Source: CAD feature listing. Evaluate the final solid. Frame: model axes, mm. Face numbers are marked on the shaded views. Round coordinates to 2 decimals unless told otherwise and drop trailing zeros. Write each loop counter-clockwise with the first axis right and the second up, starting at its lowest first coordinate (ties: lowest second). Pieces come first, ordered by that corner, then holes. Notation, with made-up numbers: M -37,71 L 1,71 A17 cw 1,84 Z; hole C -38,83.25 d7. An arc over 180 degrees is marked long. Answer in a Markdown table with one row per item. Add a question column.
Item 1: Cut plane D-D on x = -15. Return loops of the section in (y, z), and give its area (3 significant figures).
Item 2: Cut plane C-C on x = -21.75. Return loops of the section in (y, z).
Item 3: Material intervals for probe 1 along Z at (x, y) = (-17, 3.3); probe 2 along X at (y, z) = (4.3, -16); probe 3 along Z at (x, y) = (-12.75, 1.55), sorted ascending.
Item 4: Cut plane B-B on z = -15. Return loops of the section in (x, y).
Item 5: Mould query, pull axis Z, two halves, no side actions, for the marked faces 1, 2 and 3. Classes: released by +Z, released by -Z, zero draft, split by the parting line, or undercut.
Item 6: Contact query for flat-ended pins moving along their axis: pin 1 (5 mm diameter, centred on x = -22.39, z = 15.97, fed in from +Y); pin 2 (3 mm diameter, centred on y = 2.5, z = -20.5, fed in from -X). Output: stop coordinate, or through.
Item 7: Cut plane A-A on y = 4.4. Return loops of the section in (x, z), and give its area (3 significant figures).
from build123d import *

# Parameters (mm, degrees)
SKETCH_1_R          = 15.5
SKETCH_1_R_2        = 1.55
EXTRUDE_1_DEPTH     = 5
SKETCH_3_W          = 44.726871009
SKETCH_3_H          = 71.780776613
CUT_EXTRUDE_2_DEPTH = 10
FILLET_1_R          = 2
FILLET_2_R          = 5


with BuildPart() as part:
    # 草图1 → 凸台-拉伸1 (new body)
    with BuildSketch(Plane(origin=(0, 0, 0), x_dir=(1, 0, 0), z_dir=(0, 1, 0))):
        with BuildLine():
            Line((-17.783419244, 26), (17.783419244, 26))
            ThreePointArc((17.783419244, 26), (22.273863607, 22.273863607), (26, 17.783419244))
            Line((26, 17.783419244), (26, -17.783419244))
            ThreePointArc((26, -17.783419244), (22.273863607, -22.273863607), (17.783419244, -26))
            Line((17.783419244, -26), (-17.783419244, -26))
            ThreePointArc((-17.783419244, -26), (-22.273863607, -22.273863607), (-26, -17.783419244))
            Line((-26, -17.783419244), (-26, 17.783419244))
            ThreePointArc((-26, 17.783419244), (-22.273863607, 22.273863607), (-17.783419244, 26))
        make_face()
        with Locations(Location((0, 0, 0), (0, 0, 270))):
            Circle(SKETCH_1_R, mode=Mode.SUBTRACT)
        with Locations(Location((-22.388176755, 15.969331282, 0), (0, 0, 270))):
            Circle(SKETCH_1_R_2, mode=Mode.SUBTRACT)
        with Locations(Location((-15.969331282, 22.388176755, 0), (0, 0, 90))):
            Circle(SKETCH_1_R_2, mode=Mode.SUBTRACT)
        with Locations(Location((22.388176755, 15.969331282, 0), (0, 0, 90))):
            Circle(SKETCH_1_R_2, mode=Mode.SUBTRACT)
        with Locations(Location((15.969331282, 22.388176755, 0), (0, 0, 270))):
            Circle(SKETCH_1_R_2, mode=Mode.SUBTRACT)
        with Locations(Location((22.388176755, -15.969331282, 0), (0, 0, 270))):
            Circle(SKETCH_1_R_2, mode=Mode.SUBTRACT)
        with Locations(Location((15.969331282, -22.388176755, 0), (0, 0, 90))):
            Circle(SKETCH_1_R_2, mode=Mode.SUBTRACT)
        with Locations(Location((-22.388176755, -15.969331282, 0), (0, 0, 90))):
            Circle(SKETCH_1_R_2, mode=Mode.SUBTRACT)
        with Locations(Location((-15.969331282, -22.388176755, 0), (0, 0, 270))):
            Circle(SKETCH_1_R_2, mode=Mode.SUBTRACT)
    extrude(amount=EXTRUDE_1_DEPTH)

    # 草图3 → 切除-拉伸2 (cut)
    with BuildSketch(Plane(origin=(0, 5, 0), x_dir=(1, 0, 0), z_dir=(0, 1, 0))):
        with Locations((12.363435504, 5.528436561)):
            Rectangle(SKETCH_3_W, SKETCH_3_H)
    extrude(amount=-CUT_EXTRUDE_2_DEPTH, mode=Mode.SUBTRACT)

    # 圆角1
    fillet_1_edges = [part.edges().sort_by_distance(p)[0] for p in [
        (-10, 2.5, -26),
        (-10, 2.5, 26),
    ]]
    fillet(fillet_1_edges, radius=FILLET_1_R)

    # 圆角2
    fillet_2_edges = [part.edges().sort_by_distance(p)[0] for p in [
        (-17.783419244, 2.5, -26),
        (-17.783419244, 2.5, 26),
        (-26, 2.5, 17.783419244),
        (-26, 2.5, -17.783419244),
    ]]
    fillet(fillet_2_edges, radius=FILLET_2_R)


solid = part.part
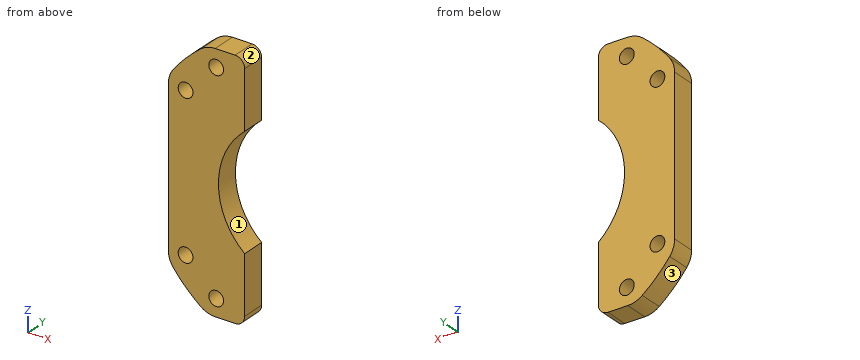
Results below:
| question | item | result |
|---|---|---|
| 1 | outline | M 0,-26 L 5,-26 L 5,-23.6 L 0,-23.6 Z; M 0,-21.18 L 5,-21.18 L 5,-3.91 L 0,-3.91 Z; M 0,3.91 L 5,3.91 L 5,21.18 L 0,21.18 Z; M 0,23.6 L 5,23.6 L 5,26 L 0,26 Z |
| 1 | area | 197 mm2 |
| 2 | outline | M 0,-22.79 L 5,-22.79 L 5,-17.38 L 0,-17.38 Z; M 0,-14.56 L 5,-14.56 L 5,14.56 L 0,14.56 Z; M 0,17.38 L 5,17.38 L 5,22.79 L 0,22.79 Z |
| 3 | probe 1 | -25.93 to -23.55, -21.23 to 21.23, 23.55 to 25.93 |
| 3 | probe 2 | -26 to -23.94, -20.84 to -10 |
| 3 | probe 3 | -26 to -8.81, 8.81 to 26 |
| 4 | outline | M -26,0 L -23.6,0 L -23.6,5 L -26,5 Z; M -21.18,0 L -10,0 L -10,5 L -21.18,5 Z |
| 5 | face 1 | undercut |
| 5 | face 2 | released by +Z |
| 5 | face 3 | released by -Z |
| 6 | pin 1 | y = 5 |
| 6 | pin 2 | x = -25.12 |
| 7 | outline | M -26,-16.16 A5 ccw -24.96,-19.21 A31.5 ccw -19.21,-24.96 A5 ccw -16.16,-26 L -12,-26 A2 ccw -10,-24 L -10,-11.84 A15.5 cw -10,11.84 L -10,24 A2 ccw -12,26 L -16.16,26 A5 ccw -19.21,24.96 A31.5 ccw -24.96,19.21 A5 ccw -26,16.16 Z; hole C -22.39,-15.97 d3.1; hole C -22.39,15.97 d3.1; hole C -15.97,-22.39 d3.1; hole C -15.97,22.39 d3.1 |
| 7 | area | 649 mm2 |
